from build123d import *

# Parameters (mm, degrees)
SKETCH2_W           = 9.84
SKETCH2_H           = 8.2
BOSS_EXTRUDE1_DEPTH = 7
SKETCH3_W           = 5.84
SKETCH3_H           = 4.2
CUT_EXTRUDE1_DEPTH  = 15.596766765
SKETCH4_R           = 4.66
BOSS_EXTRUDE2_DEPTH = 10
SKETCH5_R           = 2.66
CUT_EXTRUDE2_DEPTH  = 10


with BuildPart() as part:
    # Sketch2 → Boss-Extrude1 (new body)
    with BuildSketch(Plane(origin=(0, 0, 0), x_dir=(1, 0, 0), z_dir=(0, 1, 0))):
        with Locations((4.92, 4.1)):
            Rectangle(SKETCH2_W, SKETCH2_H)
    extrude(amount=BOSS_EXTRUDE1_DEPTH)

    # Sketch3 → Cut-Extrude1 (cut, through all)
    with BuildSketch(Plane(origin=(0, 7, 0), x_dir=(1, 0, 0), z_dir=(0, 1, 0))):
        with Locations((4.92, 4.1)):
            Rectangle(SKETCH3_W, SKETCH3_H)
    extrude(amount=-CUT_EXTRUDE1_DEPTH, mode=Mode.SUBTRACT)

    # Sketch4 → Boss-Extrude2 (add)
    with BuildSketch(Plane(origin=(0, 7, 0), x_dir=(1, 0, 0), z_dir=(0, 1, 0))):
        with Locations(Location((4.92, 4.1, 0), (0, 0, 61.621661447))):
            Circle(SKETCH4_R)
    extrude(amount=BOSS_EXTRUDE2_DEPTH)

    # Sketch5 → Cut-Extrude2 (cut)
    with BuildSketch(Plane(origin=(0, 17, 0), x_dir=(1, 0, 0), z_dir=(0, 1, 0))):
        with Locations(Location((4.92, 4.1, 0), (0, 0, 270))):
            Circle(SKETCH5_R)
    extrude(amount=-CUT_EXTRUDE2_DEPTH, mode=Mode.SUBTRACT)


solid = part.part
Design review of the part built by this model. Coordinates are the model's own, in mm. A direction names the side the tool comes from. Give positions to 0.01 mm unless a question says otherwise; leave off trailing zeros. Order: outer loops, then holes, each group sorted by start corner. A loop starts at its lowest first (then second) coordinate and runs counter-clockwise, first axis right, second up. Notation, with made-up numbers: (48.25, 59) - (57.25, 59) arc R12 ccw to (57.25, 74) - close; hole circle Ø10 at (-5.75, 18.5). An arc over 180 degrees is marked (long way). Write item = value, one per line. Start each with the question number.
Q1. Clearance check with flat-ended pins moving along their axes: pin 1 Ø2 at (x, y) = (3.5, 4.5) entering from -Z; pin 2 Ø5 at (x, z) = (4.92, -4.1) entering from +Y; pin 3 Ø5.5 at (x, y) = (3, 4) entering from +Z. State where each tip first meets the part, or that it passes through.
Q2. Tool access review of faces 4 (the face through (5, 3, 0)), 5 (the face through (5.037, 12.07, -6.757)), 6 (the face through (5, 4, -2)): name each direction out of +Z, -Z, +X, -X, +Y, -Y from which nothing blocks a thin tool from reaching the whole face with its end or side.
Q3. To check wall thickness, follow L1, parallel to Z at x = 4.92, y = 11; L2, parallel to X at y = 9.5, z = -4.1; L3, parallel to Z at x = 5.5, y = 4. State the ranges of each line that lie inside material, in increasing order. Write a range as from..to.
Q4. We need section B-B on z = -4.1. State the section outline as (x, y) points, plus the area to 3 significant figures.
Q5. We need section C-C on y = 15.5. State the section outline as (x, z) points.
Q6. We need section A-A on x = 4.92. State the section outline as (y, z) points.
Q7. We need section D-D on x = 8.5. State the section outline as (y, z) points, plus the area to 3 significant figures.
Q8. Mouldability with a two-part tool opening along X and no side actions: class faces 1 (the face through (5, 3, -8.2)), 2 (the face through (7.84, 4, -4)), 3 (the face through (0.517, 11.93, -2.575)) as released by +X, released by -X, zero draft, split by the parting line, or undercut.
Working result:
q1.pin_1 = -8.2
q1.pin_2 = 7
q1.pin_3 = 0
q2.face_4 = +Z, +X, -X, -Y
q2.face_5 = +Y
q2.face_6 = -Y
q3.L1 = -8.76..-6.76, -1.44..0.56
q3.L2 = 0.26..2.26, 7.58..9.58
q3.L3 = -8.2..-6.2, -2..0
q4.outline = (0, 0) - (2, 0) - (2, 7) - (2.26, 7) - (2.26, 17) - (0.26, 17) - (0.26, 7) - (0, 7) - close; (7.58, 7) - (7.84, 7) - (7.84, 0) - (9.84, 0) - (9.84, 7) - (9.58, 7) - (9.58, 17) - (7.58, 17) - close
q4.area = 68.0 mm²
q5.outline = circle Ø9.32 at (4.92, -4.1); hole circle Ø5.32 at (4.92, -4.1)
q6.outline = (0, -8.2) - (7, -8.2) - (7, -8.76) - (17, -8.76) - (17, -6.76) - (7, -6.76) - (7, -6.2) - (0, -6.2) - close; (0, -2) - (7, -2) - (7, -1.44) - (17, -1.44) - (17, 0.56) - (7, 0.56) - (7, 0) - (0, 0) - close
q7.outline = (0, -8.2) - (7, -8.2) - (7, -7.08) - (17, -7.08) - (17, -1.12) - (7, -1.12) - (7, 0) - (0, 0) - close
q7.area = 117 mm²
q8.face_1 = zero draft
q8.face_2 = undercut
q8.face_3 = split by the parting line
